from build123d import *

# Parameters (mm, degrees)
EXTRUDE_659_DEPTH           = 5
SKETCH_4_R                  = 3.75
CUT_EXTRUDE_1016_DEPTH      = 33.230936168
CUT_EXTRUDE_1190_REACH      = 40.468
CUT_EXTRUDE_1190_END_RADIUS = 3.75
SKETCH_5_R                  = 3.75
FILLET_8_R                  = 5


with BuildPart() as part:
    # Эскиз3 → Extrude 659 (new, symmetric)
    with BuildSketch(Plane.XY):
        Polygon((-5, 7), (-16.790187199, 16.89314173), (-10.362311102, 24.553586161), (-5, 20.054072893), (-5, 27.054072893), (5, 27.054072893), (5, 20.054072893), (10.362311102, 24.553586161), (16.790187199, 16.89314173), (5, 7), (5, 0), (-5, 0), align=None)
    extrude(amount=EXTRUDE_659_DEPTH, both=True)

    # Эскиз4 → Cut-Extrude 1016 (cut, through all)
    with BuildSketch(Plane(origin=(0, 27.054072893, 0), x_dir=(-1, 0, 0), z_dir=(0, 1, 0))):
        with Locations(Location((0, 0, 0), (0, 0, 90))):
            Circle(SKETCH_4_R)
    extrude(amount=-CUT_EXTRUDE_1016_DEPTH, mode=Mode.SUBTRACT)

    # Cut-Extrude 1190: up to this cylinder (the profile starts outside it)
    cut_extrude_1190_end = Plane(origin=(0, 20.723364, 0), z_dir=(0, 1, 0)) * Cylinder(CUT_EXTRUDE_1190_END_RADIUS, 89.436, mode=Mode.PRIVATE)
    # Эскиз5 → Cut-Extrude 1190 (cut, up to the surface)
    with BuildSketch(Plane(origin=(-18.171134778, 15.247392491, 0), x_dir=(0, 0, 1), z_dir=(-0.7660444431189745, 0.6427876096865438, 0)), mode=Mode.PRIVATE) as cut_extrude_1190_sk1:
        with Locations(Location((0, 7.148373053, 0), (0, 0, 270))):
            Circle(SKETCH_5_R)
    cut_extrude_1190_tool1 = extrude(cut_extrude_1190_sk1.sketch, amount=-CUT_EXTRUDE_1190_REACH, mode=Mode.PRIVATE) - cut_extrude_1190_end
    cut_extrude_1190 = cut_extrude_1190_tool1.solids().sort_by_distance((-13.576249, 20.723364, 0))[0]
    add(cut_extrude_1190, mode=Mode.SUBTRACT)

    # Зеркальное отражение1: Cut-Extrude 1190 across plane
    add(cut_extrude_1190.mirror(Plane(origin=(0, 0, 0), x_dir=(0, 0, 1), z_dir=(1, 0, 0))), mode=Mode.SUBTRACT)

    # Скругление8
    fillet_8_edges = [part.edges().sort_by_distance(p)[0] for p in [
        (7.681155551, 22.303829527, -5),
        (5, 23.554072893, -5),
        (-5, 23.554072893, -5),
        (-7.681155551, 22.303829527, -5),
        (-10.895093599, 11.946570865, -5),
        (-5, 3.5, -5),
        (5, 3.5, -5),
        (10.895093599, 11.946570865, -5),
        (-5, 3.5, 5),
        (5, 3.5, 5),
        (10.895093599, 11.946570865, 5),
        (7.681155551, 22.303829527, 5),
        (5, 23.554072893, 5),
        (-5, 23.554072893, 5),
        (-7.681155551, 22.303829527, 5),
        (-10.895093599, 11.946570865, 5),
    ]]
    fillet(fillet_8_edges, radius=FILLET_8_R - 0.0001)  # a hair under: the kernel refuses the full size

    # Split Bodies 2695
    split(bisect_by=Plane.XY, keep=Keep.BOTTOM)


solid = part.part
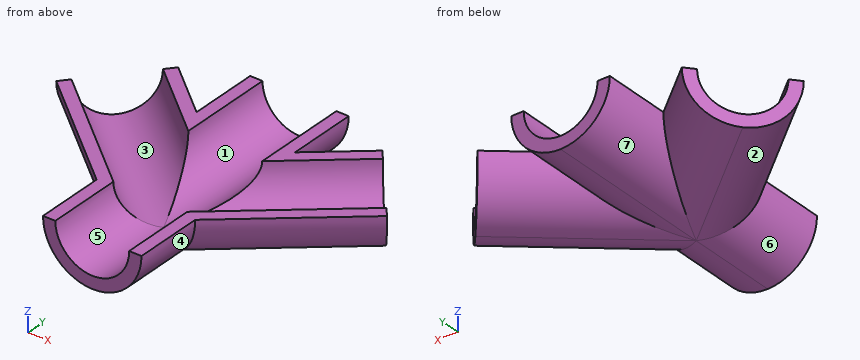
Here's how the part is built. I have some questions about the finished solid (model axes, mm). Face numbers are marked on the shaded views. A direction names the side the tool comes from. Round coordinates to 2 decimals unless told otherwise and drop trailing zeros. Order: outer loops, then holes, each group sorted by start corner. A loop starts at its lowest first (then second) coordinate and runs counter-clockwise, first axis right, second up. Notation, with made-up numbers: (54.25, 55) -> (109.25, 55) arc R28 cw to (109.25, 83) -> close; hole circle Ø1 at (-9, -3). An arc over 180 degrees is marked (long way). Return JSON: item names as keys, results as strings.
Q1. If we section it at A-A on z = -2.7: List the corners of the cut face in (x, y) for me.
Filled sheet:
{"outline": "(-16.28, 17.5) -> (-4.21, 7.37) -> (-4.21, 0) -> (-2.6, 0) -> (-2.6, 8.12) -> (-15.25, 18.73) -> close; (-11.9, 22.72) -> (-2.6, 14.91) -> (-2.6, 27.05) -> (-4.21, 27.05) -> (-4.21, 18.36) -> (-10.87, 23.95) -> close; (2.6, 0) -> (4.21, 0) -> (4.21, 7.37) -> (16.28, 17.5) -> (15.25, 18.73) -> (2.6, 8.12) -> close; (2.6, 14.91) -> (11.9, 22.72) -> (10.87, 23.95) -> (4.21, 18.36) -> (4.21, 27.05) -> (2.6, 27.05) -> close"}
Q2. If we section it at B-B on y = 21.5: Give the number of separate pieces and of enclosed holes in the cut face, plus the area to 3 significant figures.
Filled sheet:
{"separate pieces": "3", "enclosed holes": "0", "area": "39.9 mm^2"}
Q3. If we section it at D-D on z = -0.45: List the corners of the cut face in (x, y) for me.
Filled sheet:
{"outline": "(-16.78, 16.91) -> (-4.98, 7.01) -> (-4.98, 0) -> (-3.72, 0) -> (-3.72, 7.6) -> (-15.97, 17.87) -> close; (-11.18, 23.58) -> (-3.72, 17.32) -> (-3.72, 27.05) -> (-4.98, 27.05) -> (-4.98, 20.01) -> (-10.38, 24.54) -> close; (3.72, 0) -> (4.98, 0) -> (4.98, 7.01) -> (16.78, 16.91) -> (15.97, 17.87) -> (3.72, 7.6) -> close; (3.72, 17.32) -> (11.18, 23.58) -> (10.38, 24.54) -> (4.98, 20.01) -> (4.98, 27.05) -> (3.72, 27.05) -> close"}
Q4. If we mould it in two halves opening along X, with no side actions, what happens to the marked faces 1, 2, 3 and 4? For each: released by +X, released by -X, zero draft, split by the parting line, or undercut.
Filled sheet:
{"face 1": "undercut", "face 2": "released by -X", "face 3": "undercut", "face 4": "released by +X"}
Q5. I need wall thicknesses on line 1 along X through (y, z) = (20.5, -0.7); line 2 along X through (y, z) = (14.75, -2.95); line 3 along Y through (x, z) = (-9, -1.2). Which ranges of each line are inside material? Lowest first, please. Write a range as from..to.
Filled sheet:
{"line 1": "x = -7.58..-5.61, -4.95..-3.68, 3.68..4.95, 5.61..7.58", "line 2": "x = -12.74..-10.06, -2.86..-2.32, 2.32..2.86, 10.06..12.74", "line 3": "y = 10.55..12.25, 21.52..23.22"}
Q6. If we section it at C-C on z = -4.5: List the corners of the cut face in (x, y) for me, plus the area to 3 significant figures.
Filled sheet:
{"outline": "(-14.98, 19.05) -> (-2.18, 8.32) -> (-2.18, 0) -> (2.18, 0) -> (2.18, 8.32) -> (14.98, 19.05) -> (12.18, 22.39) -> (2.18, 14.01) -> (2.18, 27.05) -> (-2.18, 27.05) -> (-2.18, 14.01) -> (-12.18, 22.39) -> close", "area": "248 mm^2"}
Q7. Which directions (+Z, -Z, +X, -X, +Y, -Y) give clear straight access to the entire face, cutting with the end or side of a thin tool? Please do the marked faces 5, 6 and 7.
Filled sheet:
{"face 5": "+Z, +Y, -Y", "face 6": "-Z, -X, -Y", "face 7": "-Z, +Y"}
